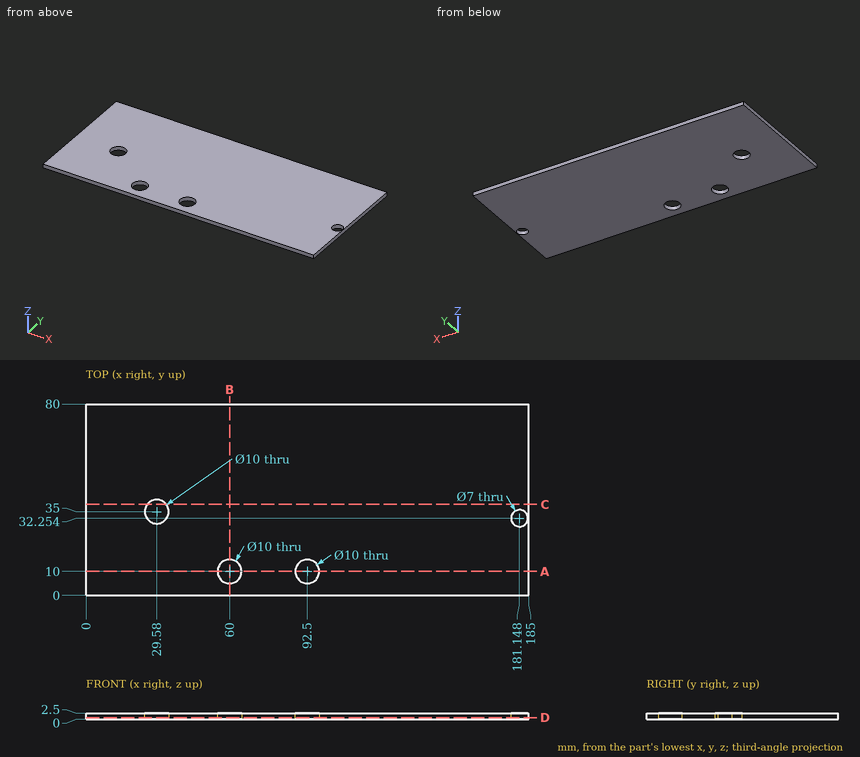
Input: dimensioned drawing with shaded views. Units: mm. Origin: part minimum x, y, z. Coordinates: 2 decimals unless noted, no trailing zeros. Loops run counter-clockwise (first coordinate to the right, second up) from the corner with the lowest first, then second, coordinate; pieces in that order, holes last. Notation, with made-up numbers: (79, 80) -> (93, 80) arc R25 ccw to (93, 112) -> close; hole circle Ø8 at (48.25, 73.5). An arc over 180 degrees is marked (long way). One line per item, written item: value. Start each with the question number.
Q1. Line query: line 1 along Y through (x, z) = (92.5, 1.75); line 2 along X through (y, z) = (32, 1.95) (1 decimal); line 3 along Y through (x, z) = (25.5, 0.3). Output: solid intervals per line, ascending.
Q2. Contact query for flat-ended pins moving along their axis: P1, Ø8, axis at x = 29.58, y = 35, coming from the -Z side; P2, Ø11, axis at x = 181.15, y = 32.25, coming from the -Z side. Output: stop coordinate, or through.
Q3. Section query D-D, the plane z = 0.75. Return the cut outline in (x, y) (1 decimal).
Q4. Section query C-C, the plane y = 38. Return the cut outline in (x, z).
Q5. Section query A-A, the plane y = 10. Return the cut outline in (x, z).
Q6. Section query B-B, the plane x = 60. Return the cut outline in (y, z).
Results:
1. line 1: 0 to 5, 15 to 80
1. line 2: 0 to 25.6, 33.6 to 177.7, 184.6 to 185
1. line 3: 0 to 32.11, 37.89 to 80
2. P1: through
2. P2: z = 0
3. outline: (0, 0) -> (185, 0) -> (185, 80) -> (0, 80) -> close; hole circle Ø10 at (29.6, 35); hole circle Ø10 at (60, 10); hole circle Ø10 at (92.5, 10); hole circle Ø7 at (181.1, 32.3)
4. outline: (0, 0) -> (25.58, 0) -> (25.58, 2.5) -> (0, 2.5) -> close; (33.58, 0) -> (185, 0) -> (185, 2.5) -> (33.58, 2.5) -> close
5. outline: (0, 0) -> (55, 0) -> (55, 2.5) -> (0, 2.5) -> close; (65, 0) -> (87.5, 0) -> (87.5, 2.5) -> (65, 2.5) -> close; (97.5, 0) -> (185, 0) -> (185, 2.5) -> (97.5, 2.5) -> close
6. outline: (0, 0) -> (5, 0) -> (5, 2.5) -> (0, 2.5) -> close; (15, 0) -> (80, 0) -> (80, 2.5) -> (15, 2.5) -> close
